For this review, use the dimensioned drawing (mm, ordinates from the lowest corner) and the shaded views. A direction names the side the tool comes from. Coordinates: 2 decimals unless noted, no trailing zeros. Write each loop counter-clockwise with the first axis right and the second up, starting at its lowest first coordinate (ties: lowest second). Pieces come first, ordered by that corner, then holes. Notation, with made-up numbers: (11.5, 2.5) - (19.5, 2.5) arc R24 ccw to (19.5, 13.5) - close; hole circle Ø1 at (-17, -37). An arc over 180 degrees is marked (long way). Put each result on its own line as item: value.
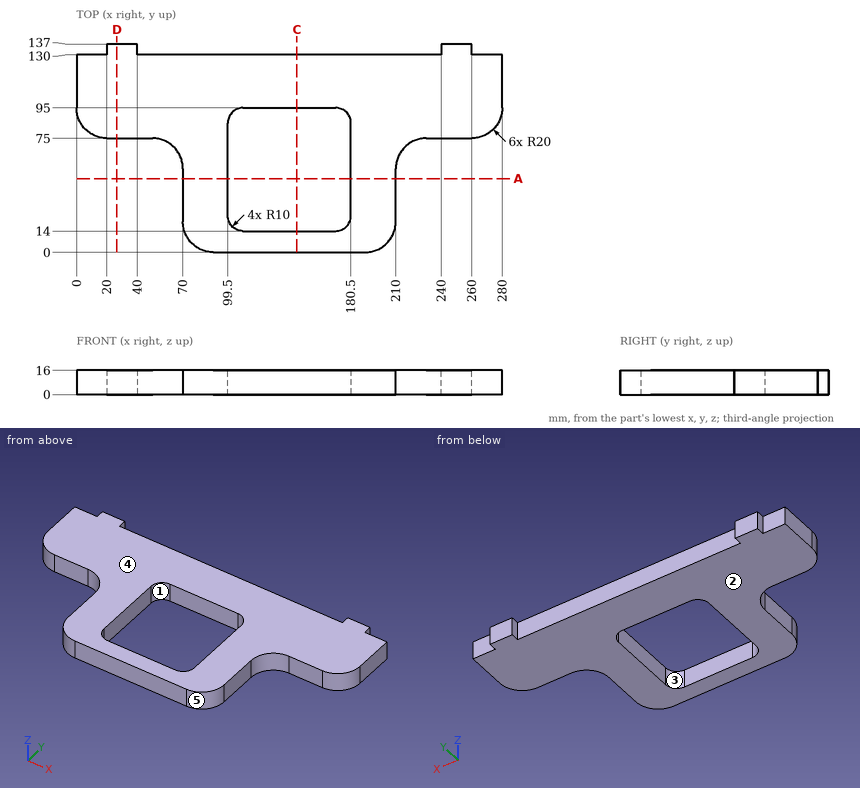
1. The part is to be moulded in two halves that separate along X. For the marked faces 3, 4 and 5, say which applies: +X half, -X half, draft (parallel to the pull), parting line (faces both ways), or undercut.
Determined:
face 3: undercut
face 4: draft
face 5: +X half
2. Machinability: for the marked faces 1 and 2, which of the approach directions +Z, -Z, +X, -X, +Y, -Y give a long, thin tool a straight path to every point of the face, cutting with its end or side? Answer none if there is none.
Determined:
face 1: +Z, -Z
face 2: -Z, +X, -X, +Y, -Y
3. Consider section A-A on y = 48.5. State the section outline as (x, z) points, plus the area to 3 significant figures.
Determined:
outline: (70, 0) - (99.5, 0) - (99.5, 16) - (70, 16) - close; (180.5, 0) - (210, 0) - (210, 16) - (180.5, 16) - close
area: 944 mm^2
4. For pin 1 Ø6 at (x, y) = (207.5, 92.5) entering from -Z; pin 2 Ø7.5 at (y, z) = (134.5, 8) entering from -X; pin 3 Ø8 at (y, z) = (69, 4.5) entering from +X; pin 4 Ø3.5 at (y, z) = (133, 6.5) entering from +X, all flat-tipped, find the tip position at first contact; note any pin that passes through.
Determined:
pin 1: stops at z = 0
pin 2: stops at x = 20
pin 3: stops at x = 221.28
pin 4: stops at x = 260
5. Consider section D-D on x = 26.5. State the section outline as (y, z) points, plus the area to 3 significant figures.
Determined:
outline: (75, 0) - (137, 0) - (137, 16) - (75, 16) - close
area: 992 mm^2
6. To check wall thickness, follow probe 1 along X at (y, z) = (54, 14.5); probe 2 along Y at (x, z) = (134, 2.5); probe 3 along X at (y, z) = (69.5, 6). State the ranges of each line that lie inside material, in increasing order.
Determined:
probe 1: x = 70 to 99.5, 180.5 to 210
probe 2: y = 0 to 14, 95 to 130
probe 3: x = 63.77 to 99.5, 180.5 to 216.23
7. Consider section C-C on x = 145. State the section outline as (y, z) points, plus the area to 3 significant figures.
Determined:
outline: (0, 0) - (14, 0) - (14, 16) - (0, 16) - close; (95, 0) - (130, 0) - (130, 16) - (95, 16) - close
area: 784 mm^2
